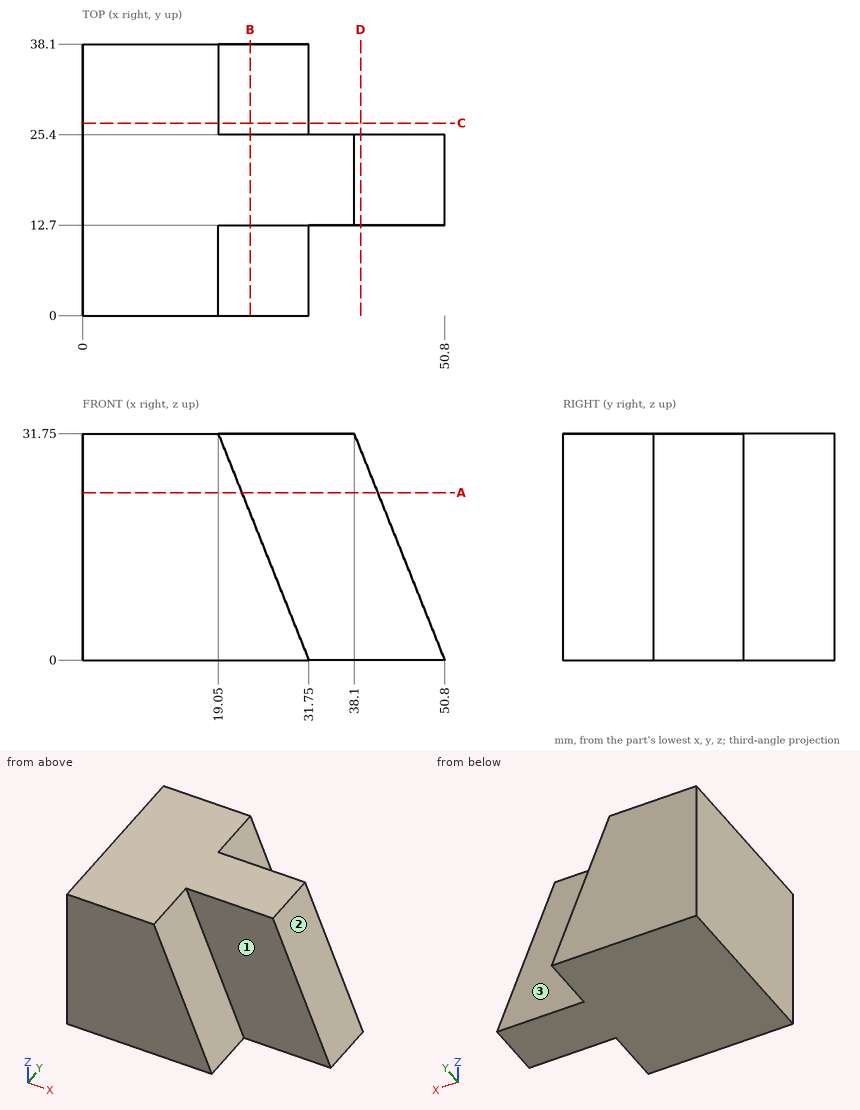
Input: dimensioned drawing with shaded views. Units: mm. Origin: part minimum x, y, z. A direction names the side the tool comes from. Coordinates: 2 decimals unless noted, no trailing zeros. Loops run counter-clockwise (first coordinate to the right, second up) from the corner with the lowest first, then second, coordinate; pieces in that order, holes last.
Q1. Section A-A, the plane z = 23.5. Return the cut outline in (x, y).
Results are:
outline: (0, 0) - (22.35, 0) - (22.35, 12.7) - (41.4, 12.7) - (41.4, 25.4) - (22.35, 25.4) - (22.35, 38.1) - (0, 38.1) - close
Q2. Contact query for a flat-ended pin moving along its axis: pin 1 (2 mm diameter, centred on x = 22.5, y = 7, fed in from +Z) (3 decimals). Output: stop coordinate, or through.
Results are:
pin 1: stops at z = 25.625
Q3. Set-up query: the marked faces 1, 2 and 3. Return all of +Z, -Z, +X, -X, +Y, -Y with unobstructed straight access to the full face (end or side cutting, diameter ignored); none if empty.
Results are:
face 1: +Z, +X, -Y
face 2: +Z, +X, +Y, -Y
face 3: +Z, +X, +Y
Q4. Line query: line 1 along Y through (x, z) = (38.5, 4); line 2 along X through (y, z) = (29.5, 14); line 3 along X through (y, z) = (34, 4.5). Output: solid intervals per line, ascending.
Results are:
line 1: y = 12.7 to 25.4
line 2: x = 0 to 26.15
line 3: x = 0 to 29.95
Q5. Section C-C, the plane y = 27. Return the cut outline in (x, z), and give its area (3 significant figures).
Results are:
outline: (0, 0) - (31.75, 0) - (19.05, 31.75) - (0, 31.75) - close
area: 806 mm2
Q6. Section B-B, the plane x = 23.5. Return the cut outline in (y, z) (3 decimals), and give its area (3 significant figures).
Results are:
outline: (0, 0) - (38.1, 0) - (38.1, 20.625) - (25.4, 20.625) - (25.4, 31.75) - (12.7, 31.75) - (12.7, 20.625) - (0, 20.625) - close
area: 927 mm2
Q7. Section D-D, the plane x = 39. Return the cut outline in (y, z), and give its area (3 significant figures).
Results are:
outline: (12.7, 0) - (25.4, 0) - (25.4, 29.5) - (12.7, 29.5) - close
area: 375 mm2
